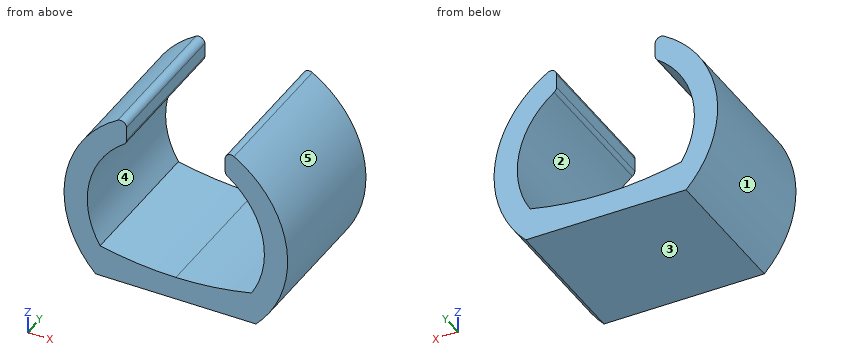
from build123d import *

# Parameters (mm, degrees)
F1_DEPTH = 25
F2_W     = 17
F2_H     = 6.5885427379
F3_DEPTH = 25.001
F4_R     = 1
F6_DEPTH = 25


with BuildPart() as f1:
    # F0 (on Front) → F1 (new body)
    with BuildSketch(Plane.XZ):
        with BuildLine():
            Line((-13.8099195907, -13.4107651124), (13.8099195907, -13.4107651124))
            ThreePointArc((13.8099195907, -13.4107651124), (0, 19.25), (-13.8099195907, -13.4107651124))
        make_face()
        with BuildLine():
            ThreePointArc((-12, -9.4107651124), (0, 15.25), (12, -9.4107651124))
            Line((12, -9.4107651124), (-12, -9.4107651124))
        make_face(mode=Mode.SUBTRACT)
    extrude(amount=F1_DEPTH)

    # F2 (on face) → F3 (cut, through all)
    with BuildSketch(Plane.XZ.offset(25)):
        with Locations((0, 15.9557286311)):
            Rectangle(F2_W, F2_H)
    extrude(amount=-F3_DEPTH, mode=Mode.SUBTRACT)

    # F4
    f4_edges = [f1.edges().sort_by_distance(p)[0] for p in [
        (-8.5, -12.5, 17.271725),
        (-8.5, -12.5, 12.661457),
        (8.5, -12.5, 17.271725),
        (8.5, -12.5, 12.661457),
    ]]
    fillet(f4_edges, radius=F4_R)

    # F5 (on face) → F6 (join, through all)
    with BuildSketch(Plane.XZ.offset(25)):
        with BuildLine():
            ThreePointArc((13.0377258499, -7.9107651124), (6.5618652017, -9.0345323104), (1.674e-07, -9.4107651124))
            Line((1.674e-07, -9.4107651124), (12, -9.4107651124))
            ThreePointArc((12, -9.4107651124), (12.5413089003, -8.6762936249), (13.0377258499, -7.9107651124))
        make_face()
        with BuildLine():
            ThreePointArc((1.674e-07, -9.4107651124), (-6.5618650354, -9.0345323295), (-13.0377258499, -7.9107651124))
            ThreePointArc((-13.0377258499, -7.9107651124), (-12.5413089003, -8.6762936249), (-12, -9.4107651124))
            Line((-12, -9.4107651124), (1.674e-07, -9.4107651124))
        make_face()
    extrude(amount=-F6_DEPTH)


solid = f1.part
Source: CAD feature listing. Evaluate the final solid. Frame: model axes, mm. Face numbers are marked on the shaded views. A direction names the side the tool comes from. Coordinates: 2 decimals unless noted, no trailing zeros. Order: outer loops, then holes, each group sorted by start corner. A loop starts at its lowest first (then second) coordinate and runs counter-clockwise, first axis right, second up.
Item 1: Material intervals for line 1 (X direction, y = -7.5, z = -0.5); line 2 (X direction, y = -15.25, z = 11.25); line 3 (Z direction, x = -10, y = -19), sorted ascending.
Output values:
line 1: x = -19.24 to -15.24, 15.24 to 19.24
line 2: x = -15.62 to -10.3, 10.3 to 15.62
line 3: z = -13.41 to -8.53, 11.51 to 16.45
Item 2: Cut plane A-A (z = -2.25). Return loops of the section in (x, y).
Output values:
outline: (-19.12, -25) - (-15.08, -25) - (-15.08, 0) - (-19.12, 0) - close; (15.08, -25) - (19.12, -25) - (19.12, 0) - (15.08, 0) - close
Item 3: First-contact query: P1, Ø2.5, axis at y = -17.5, z = 15, coming from the +X side; P2, Ø10, axis at y = -18.5, z = 10, coming from the +X side; P3, Ø1.5, axis at x = 12, y = -13, coming from the +Z side. Flat tips, straight axial feed; report the tip coordinate or a pass-through.
Output values:
P1: stops at x = 13.47
P2: stops at x = 18.59
P3: stops at z = 15.62
Item 4: Set-up query: the marked faces 1 and 2. Return all of +Z, -Z, +X, -X, +Y, -Y with unobstructed straight access to the full face (end or side cutting, diameter ignored); none if empty.
Output values:
face 1: -X, +Y, -Y
face 2: +Y, -Y
Item 5: Pull-direction query (Z, two-part tool) for the marked faces 3, 4 and 5; classes: pulls with the +Z half, pulls with the -Z half, needs draft (parallel to the pull), parting line crosses it, or undercut.
Output values:
face 3: pulls with the -Z half
face 4: undercut
face 5: parting line crosses it
Item 6: Cut plane D-D (x = 5). Return loops of the section in (y, z), plus the area to 3 significant figures.
Output values:
outline: (-25, -13.41) - (0, -13.41) - (0, -9.19) - (-25, -9.19) - close
area: 105 mm2
Item 7: Cut plane C-C (y = -6.5). Return loops of the section in (x, z).
Output values:
outline: (-13.81, -13.41) - (13.81, -13.41) arc R19.25 ccw to (10.02, 16.44) arc R1 ccw to (8.5, 15.58) - (8.5, 13.18) arc R1 ccw to (8.92, 12.37) arc R15.25 cw to (13.04, -7.91) arc R57.41 cw to (-13.04, -7.91) arc R15.25 cw to (-8.92, 12.37) arc R1 ccw to (-8.5, 13.18) - (-8.5, 15.58) arc R1 ccw to (-10.02, 16.44) arc R19.25 ccw to start
Item 8: Cut plane B-B (x = -12). Return loops of the section in (y, z).
Output values:
outline: (-25, -13.41) - (0, -13.41) - (0, -8.14) - (-25, -8.14) - close; (-25, 9.41) - (0, 9.41) - (0, 15.05) - (-25, 15.05) - close
